from build123d import *

# Parameters (mm, degrees)
SKETCH_1_R      = 44
SKETCH_1_R_2    = 1.525
SKETCH_1_R_3    = 11.025
SKETCH_1_R_4    = 2
EXTRUDE_1_DEPTH = 3


with BuildPart() as part:
    # 草图1 → 凸台-拉伸1 (new body)
    with BuildSketch(Plane(origin=(0, 0, 0), x_dir=(1, 0, 0), z_dir=(0, 1, 0))):
        with Locations(Location((0, 0, 0), (0, 0, 270))):
            Circle(SKETCH_1_R)
        with Locations(Location((37, 0, 0), (0, 0, 270))):
            Circle(SKETCH_1_R_2, mode=Mode.SUBTRACT)
        with Locations(Location((18.5, -32.04293994, 0), (0, 0, 270))):
            Circle(SKETCH_1_R_2, mode=Mode.SUBTRACT)
        with Locations(Location((-18.5, -32.04293994, 0), (0, 0, 270))):
            Circle(SKETCH_1_R_2, mode=Mode.SUBTRACT)
        with Locations(Location((-37, 0, 0), (0, 0, 270))):
            Circle(SKETCH_1_R_2, mode=Mode.SUBTRACT)
        with Locations(Location((-18.5, 32.04293994, 0), (0, 0, 270))):
            Circle(SKETCH_1_R_2, mode=Mode.SUBTRACT)
        with Locations(Location((18.5, 32.04293994, 0), (0, 0, 270))):
            Circle(SKETCH_1_R_2, mode=Mode.SUBTRACT)
        with Locations(Location((0, 0, 0), (0, 0, 270))):
            Circle(SKETCH_1_R_3, mode=Mode.SUBTRACT)
        with Locations(Location((0, 20, 0), (0, 0, 270))):
            Circle(SKETCH_1_R_2, mode=Mode.SUBTRACT)
        with Locations(Location((17.320508076, -10, 0), (0, 0, 270))):
            Circle(SKETCH_1_R_2, mode=Mode.SUBTRACT)
        with Locations(Location((-17.320508076, -10, 0), (0, 0, 270))):
            Circle(SKETCH_1_R_2, mode=Mode.SUBTRACT)
        with Locations(Location((17.320508076, 10, 0), (0, 0, 270))):
            Circle(SKETCH_1_R_4, mode=Mode.SUBTRACT)
    extrude(amount=EXTRUDE_1_DEPTH)


solid = part.part
Read the model definition and answer for the solid it produces. Units are mm, in the model's axes. Round coordinates to 2 decimals unless told otherwise and drop trailing zeros. Loops run counter-clockwise (first coordinate to the right, second up) from the corner with the lowest first, then second, coordinate; pieces in that order, holes last. Notation, with made-up numbers: (45.5, 14.25) - (99.5, 14.25) arc R10 cw to (99.5, 30.25) - close; hole circle Ø1 at (-25.75, 15.25). An arc over 180 degrees is marked (long way). One line per question, with ' | ' between items. Start each with the question number.
Q1. Find the intervals of material crossed by L1, parallel to X at y = 2, z = 0 (3 decimals); L2, parallel to X at y = 2.05, z = -10; L3, parallel to Z at x = -6.5, y = 2.15, in increasing order.
Q2. Section B-B on x = -37 is taken. Give the vertices of the cut face in (y, z) (3 decimals), plus the area to 3 significant figures.
Q3. For a pull along X with two mould halves and no side action, classify faces 1 (the cylindrical face through (-42.954, 1.479, -9.538)), 2 (the flat face through (-9, 0, 9)), 3 (the cylindrical face through (35.51, 1.48, -0.33)) as +X half, -X half, draft (parallel to the pull), parting line (faces both ways), or undercut.
Q4. Section C-C on y = 0.9 is taken. Count the separate pieces of the cut face and the enclosed holes in it, plus the area to 3 significant figures.
Q5. Flat-ended cylindrical pins translate along their axes: pin 1 (8 mm diameter, centred on x = -33, z = -9.5, fed in from -Y); pin 2 (1.8 mm diameter, centred on x = 18.5, z = 32.04, fed in from -Y); pin 3 (1 mm diameter, centred on y = 1, z = -6, fed in from +X); pin 4 (1 mm diameter, centred on x = -8.5, y = 2.5, fed in from +Z). Find the tip coordinate at first contact, or state that the pin passes through.
Q6. Section D-D on z = -20 is taken. Give the vertices of the cut face in (x, y) (3 decimals).
Q7. Section A-A on z = 0 is taken. Give the vertices of the cut face in (x, y) (3 decimals), plus the area to 3 significant figures.
Established:
1) L1: -44 to -38.525, -35.475 to -11.025, 11.025 to 35.475, 38.525 to 44 | L2: -42.85 to -4.64, 4.64 to 15.32, 19.32 to 42.85 | L3: -43.52 to -8.91, 8.91 to 43.52
2) outline: (0, -23.812) - (3, -23.812) - (3, -1.525) - (0, -1.525) - close; (0, 1.525) - (3, 1.525) - (3, 23.812) - (0, 23.812) - close | area: 134 mm²
3) face 1: parting line | face 2: draft | face 3: undercut
4) separate pieces: 1 | enclosed holes: 11 | area: 5,620 mm²
5) pin 1: y = 0 | pin 2: through | pin 3: x = 43.65 | pin 4: z = 43.27
6) outline: (-39.192, 0) - (-1.525, 0) - (-1.525, 3) - (-39.192, 3) - close; (1.525, 0) - (39.192, 0) - (39.192, 3) - (1.525, 3) - close
7) outline: (-44, 0) - (-38.525, 0) - (-38.525, 3) - (-44, 3) - close; (-35.475, 0) - (-11.025, 0) - (-11.025, 3) - (-35.475, 3) - close; (11.025, 0) - (35.475, 0) - (35.475, 3) - (11.025, 3) - close; (38.525, 0) - (44, 0) - (44, 3) - (38.525, 3) - close | area: 180 mm²
